from build123d import *

# Parameters (mm, degrees)
F0_W      = 10
F0_H      = 75
F1_DEPTH  = 60
F3_DEPTH  = 330
F5_DEPTH  = 330
F7_DEPTH  = 330
F8_R      = 8
F9_DEPTH  = 25
F10_R     = 8
F11_DEPTH = 25


with BuildPart() as f1:
    # F0 (on Front) → F1 (new body)
    with BuildSketch(Plane.XZ):
        Polygon((248.9711431703, 32.5), (210, 10), (165, 10), (155, 10), (0, 10), (0, 0), (212.6794919243, 0), (524.7595264192, 180.1794919243), (524.7595264192, 40), (534.7595264192, 40), (534.7595264192, 197.5), (526.0992723813, 192.5), (257.6313972081, 37.5), align=None)
        Polygon((211.4711431703, 97.4519052838), (248.9711431703, 32.5), (257.6313972081, 37.5), (220.1313972081, 102.4519052838), align=None)
        with Locations((160, 47.5)):
            Rectangle(F0_W, F0_H)
        Polygon((488.5992723813, 257.4519052838), (526.0992723813, 192.5), (534.7595264192, 197.5), (497.2595264192, 262.4519052838), align=None)
        Polygon((0, 0), (0, 10), (-155, 10), (-165, 10), (-210, 10), (-248.9711431703, 32.5), (-257.6313972081, 37.5), (-526.0992723813, 192.5), (-534.7595264192, 197.5), (-534.7595264192, 40), (-524.7595264192, 40), (-524.7595264192, 180.1794919243), (-212.6794919243, 0), align=None)
        with Locations((-160, 47.5)):
            Rectangle(F0_W, F0_H)
        Polygon((-257.6313972081, 37.5), (-248.9711431703, 32.5), (-211.4711431703, 97.4519052838), (-220.1313972081, 102.4519052838), align=None)
        Polygon((-497.2595264192, 262.4519052838), (-534.7595264192, 197.5), (-526.0992723813, 192.5), (-488.5992723813, 257.4519052838), align=None)
    extrude(amount=F1_DEPTH)

    # F2 (on face) → F3 (cut, through all)
    with BuildSketch(Plane(origin=(-486.5896534381, 0, 280.9326673974), x_dir=(0, -1, 0), z_dir=(-0.8660254038, 0, 0.5))):
        with BuildLine():
            Line((40, -21.3397459622), (20, -21.3397459622))
            Line((20, -21.3397459622), (20, -36.3397459622))
            ThreePointArc((20, -36.3397459622), (30, -46.3397459622), (40, -36.3397459622))
            Line((40, -36.3397459622), (40, -21.3397459622))
        make_face()
    extrude(amount=-F3_DEPTH, mode=Mode.SUBTRACT)

    # F4 (on face) → F5 (cut, through all)
    with BuildSketch(Plane(origin=(-165, 0, 0), x_dir=(0, -1, 0), z_dir=(-1, 0, 0))):
        with BuildLine():
            Line((40, 70), (40, 85))
            Line((40, 85), (20, 85))
            Line((20, 85), (20, 70))
            ThreePointArc((20, 70), (30, 60), (40, 70))
        make_face()
    extrude(amount=-F5_DEPTH, mode=Mode.SUBTRACT)

    # F6 (on face) → F7 (cut, through all)
    with BuildSketch(Plane(origin=(486.5896534381, 0, 280.9326673974), x_dir=(0, 1, 0), z_dir=(0.8660254038, 0, 0.5))):
        with BuildLine():
            Line((-40, -21.3397459622), (-40, -36.3397459622))
            ThreePointArc((-40, -36.3397459622), (-30, -46.3397459622), (-20, -36.3397459622))
            Line((-20, -36.3397459622), (-20, -21.3397459622))
            Line((-20, -21.3397459622), (-40, -21.3397459622))
        make_face()
    extrude(amount=-F7_DEPTH, mode=Mode.SUBTRACT)

    # F8 (on face) → F9 (cut)
    with BuildSketch(Plane(origin=(-534.7595264192, 0, 0), x_dir=(0, -1, 0), z_dir=(-1, 0, 0))):
        with Locations((30, 60)):
            Circle(F8_R)
        with Locations((30, 120)):
            Circle(F8_R)
        with Locations((30, 90)):
            Circle(F8_R)
    extrude(amount=-F9_DEPTH, mode=Mode.SUBTRACT)

    # F10 (on face) → F11 (cut)
    with BuildSketch(Plane.YZ.offset(534.7595264192)):
        with Locations((-30, 60)):
            Circle(F10_R)
        with Locations((-30, 120)):
            Circle(F10_R)
        with Locations((-30, 90)):
            Circle(F10_R)
    extrude(amount=-F11_DEPTH, mode=Mode.SUBTRACT)


solid = f1.part
Part model, mm, in its own coordinate system. A direction names the side the tool comes from. Round coordinates to 2 decimals unless told otherwise and drop trailing zeros. Write each loop counter-clockwise with the first axis right and the second up, starting at its lowest first coordinate (ties: lowest second). Pieces come first, ordered by that corner, then holes. Notation, with made-up numbers: M 49,48.25 L 80,48.25 A16 ccw 80,77.25 Z; hole C -10,80.25 d1. An arc over 180 degrees is marked long. Return JSON: item names as keys, results as strings. Group by question number.
(1) Drill centre lines: probe 1 along X at (y, z) = (-47, 25.5); probe 2 along Z at (x, y) = (-531, -30); probe 3 along Z at (x, y) = (-532, -30). Where is each one in solid material? Low to high.
(2) Saw through at C-C on x = 41. Write the cut outline in (y, z), then the cut area to 3 significant figures.
(3) Saw through at A-A on z = 147.5. Write the cut outline in (x, y), then the cut area to 3 significant figures.
(4) Two-plate mould, pull along X, no slides. Class faces 4 (the face through (516.272, -29.58, 229.521)), 5 (the face through (155, -30, 47)), 6 (the face through (-165, -30, 47)), 7 (the face through (-2, 0, 5)): +X half, -X half, draft (parallel to the pull), parting line (faces both ways), or undercut.
(5) Saw through at B-B on z = 207. Write the cut outline in (x, y), then the cut area to 3 significant figures.
(6) Which spindle directions (+Z, -Z, +X, -X, +Y, -Y) get a long thin tool onto all of the face, cutting with end or side? Do faces 1 (the face through (-155, -30, 47)), 2 (the face through (-370.9, -29.58, 91.35)), 3 (the face through (507.087, -29.58, 225.431)). Say none if no direction does.
(7) Pin check, flat tips, straight feed: pin 1 Ø8 at (x, y) = (160, -5) entering from +Z; pin 2 Ø8 at (x, y) = (-254.5, -41.5) entering from +Z; pin 3 Ø18.5 at (y, z) = (-30, 120) entering from -X; pin 4 Ø13.5 at (x, y) = (-190.5, -34) entering from +Z. Stop position of each tip, or through.
Returned:
{
 "1": {"probe 1": "-256.85 to -236.85, -165 to -155, 155 to 165, 236.85 to 256.85", "probe 2": "40 to 52, 68 to 82, 98 to 112, 128 to 204.01", "probe 3": "40 to 52, 68 to 82, 98 to 112, 128 to 202.28"},
 "2": {"outline": "M -60,0 L 0,0 L 0,10 L -60,10 Z", "area": "600 mm²"},
 "3": {"outline": "M -534.76,-60 L -524.76,-60 L -524.76,0 L -534.76,0 Z; M -468.16,-60 L -448.16,-60 L -448.16,0 L -468.16,0 Z; M 448.16,-60 L 468.16,-60 L 468.16,0 L 448.16,0 Z; M 524.76,-60 L 534.76,-60 L 534.76,0 L 524.76,0 Z", "area": "3,600 mm²"},
 "4": {"face 4": "+X half", "face 5": "undercut", "face 6": "undercut", "face 7": "draft"},
 "5": {"outline": "M -529.27,-60 L -517.73,-60 L -517.73,0 L -529.27,0 Z; M 517.73,-60 L 529.27,-60 L 529.27,0 L 517.73,0 Z", "area": "1,390 mm²"},
 "6": {"face 1": "+Z, +Y, -Y", "face 2": "-Z, +Y, -Y", "face 3": "+Y, -Y"},
 "7": {"pin 1": "z = 85", "pin 2": "z = 49.85", "pin 3": "x = -534.76", "pin 4": "z = 10"}
}
